from build123d import *

# Parameters (mm, degrees)
SKETCH1_W             = 110
SKETCH1_H             = 46
BOSS_EXTRUDE1_DEPTH   = 6.35
F_8_CLEARANCE_HOLE2_D = 4.3053
FILLET1_R             = 5
M5_CLEARANCE_HOLE1_D  = 5.3
F_8_CLEARANCE_HOLE1_D = 4.3053
SKETCH13_R            = 2.15265
CUT_EXTRUDE2_DEPTH    = 10
CUT_EXTRUDE3_DEPTH    = 7.35


with BuildPart() as part:
    # Sketch1 → Boss-Extrude1 (new body)
    with BuildSketch(Plane.XY):
        Rectangle(SKETCH1_W, SKETCH1_H)
    extrude(amount=BOSS_EXTRUDE1_DEPTH)

    # #8 Clearance Hole2 (through all)
    with Locations(Plane(origin=(0, 0, 0), x_dir=(-1, 0, 0), z_dir=(0, 0, -1))):
        with Locations((-47, 9), (-23, 9), (-23, -9), (-47, -9), (23, -9), (23, 9), (47, 9), (47, -9)):
            Hole(F_8_CLEARANCE_HOLE2_D / 2)

    # Fillet1
    fillet1_edges = [part.edges().sort_by_distance(p)[0] for p in [
        (-55, -23, 3.175),
        (-55, 23, 3.175),
        (55, 23, 3.175),
        (55, -23, 3.175),
    ]]
    fillet(fillet1_edges, radius=FILLET1_R)

    # M5 Clearance Hole1 (through all)
    with Locations(Plane.XY.offset(6.35)):
        with Locations((-10, -5), (10, -5)):
            Hole(M5_CLEARANCE_HOLE1_D / 2)

    # #8 Clearance Hole1 (through all)
    with Locations(Plane.XY.offset(6.35)):
        with Locations((-23, 19), (-23, -19), (23, -19), (23, 19), (-50, 19), (-50, -19), (50, -19), (50, 19)):
            Hole(F_8_CLEARANCE_HOLE1_D / 2)

    # Sketch13 → Cut-Extrude2 (cut)
    with BuildSketch(Plane.XY.offset(6.35)):
        with Locations((47, 9)):
            Circle(SKETCH13_R)
        with Locations((23, -9)):
            Circle(SKETCH13_R)
        with Locations((23, 9)):
            Circle(SKETCH13_R)
        with Locations((47, -9)):
            Circle(SKETCH13_R)
        with BuildLine():
            Line((42, 10), (42, -10))
            ThreePointArc((42, -10), (35, -17), (28, -10))
            Line((28, -10), (28, 10))
            ThreePointArc((28, 10), (35, 17), (42, 10))
        make_face()
        with BuildLine():
            Line((-42, 10), (-42, -10))
            ThreePointArc((-42, -10), (-35, -17), (-28, -10))
            Line((-28, -10), (-28, 10))
            ThreePointArc((-28, 10), (-35, 17), (-42, 10))
        make_face()
    extrude(amount=-CUT_EXTRUDE2_DEPTH, mode=Mode.SUBTRACT)

    # Sketch14 → Cut-Extrude3 (cut, through all)
    with BuildSketch(Plane.XY.offset(6.35)):
        with BuildLine():
            Line((-12.5, -11), (12.5, -11))
            ThreePointArc((12.5, -11), (16.5, -15), (12.5, -19))
            Line((12.5, -19), (-12.5, -19))
            ThreePointArc((-12.5, -19), (-16.5, -15), (-12.5, -11))
        make_face()
        with BuildLine():
            Line((-12.5, 19), (12.5, 19))
            ThreePointArc((12.5, 19), (16.5, 15), (12.5, 11))
            Line((12.5, 11), (-12.5, 11))
            ThreePointArc((-12.5, 11), (-16.5, 15), (-12.5, 19))
        make_face()
    extrude(amount=-CUT_EXTRUDE3_DEPTH, mode=Mode.SUBTRACT)


solid = part.part
The listing builds one solid part. Answer for the finished solid, in the listing's coordinates (mm). A direction names the side the tool comes from. Coordinates: 2 decimals unless noted, no trailing zeros. Loops run counter-clockwise (first coordinate to the right, second up) from the corner with the lowest first, then second, coordinate; pieces in that order, holes last. Notation, with made-up numbers: M -22,-20.75 L -10,-20.75 A23 cw -10,2.25 Z; hole C 0.5,-17 d10. An arc over 180 degrees is marked long. Answer in a Markdown table with one row per item.
1) Determine the mould class of faces 1 (the flat face through (-1, 0, 6.35)), 2 (the cylindrical face through (-54, -21, 3)), 3 (the flat face through (0, -11, 3)), 4 (the cylindrical face through (-16.5, -15.1, 3.2)) for opening direction X: released by +X, released by -X, zero draft, split by the parting line, or undercut.
Answers below:
| item | result |
|---|---|
| face 1 | zero draft |
| face 2 | released by -X |
| face 3 | undercut |
| face 4 | undercut |
2) Find section A-A (x = 35). Determine the outline of the cut face in (y, z).
Answers below:
| item | result |
|---|---|
| outline | M -23,0 L -17,0 L -17,6.35 L -23,6.35 Z; M 17,0 L 23,0 L 23,6.35 L 17,6.35 Z |
3) Find section D-D (y = -14). Determine the outline of the cut face in (x, z).
Answers below:
| item | result |
|---|---|
| outline | M -55,0 L -40.74,0 L -40.74,6.35 L -55,6.35 Z; M -29.26,0 L -16.37,0 L -16.37,6.35 L -29.26,6.35 Z; M 16.37,0 L 29.26,0 L 29.26,6.35 L 16.37,6.35 Z; M 40.74,0 L 55,0 L 55,6.35 L 40.74,6.35 Z |
4) Find section C-C (y = -5). Determine the outline of the cut face in (x, z).
Answers below:
| item | result |
|---|---|
| outline | M -55,0 L -42,0 L -42,6.35 L -55,6.35 Z; M -28,0 L -12.65,0 L -12.65,6.35 L -28,6.35 Z; M -7.35,0 L 7.35,0 L 7.35,6.35 L -7.35,6.35 Z; M 12.65,0 L 28,0 L 28,6.35 L 12.65,6.35 Z; M 42,0 L 55,0 L 55,6.35 L 42,6.35 Z |
5) Find section B-B (x = -23). Determine the outline of the cut face in (y, z).
Answers below:
| item | result |
|---|---|
| outline | M -23,0 L -21.15,0 L -21.15,6.35 L -23,6.35 Z; M -16.85,0 L -11.15,0 L -11.15,6.35 L -16.85,6.35 Z; M -6.85,0 L 6.85,0 L 6.85,6.35 L -6.85,6.35 Z; M 11.15,0 L 16.85,0 L 16.85,6.35 L 11.15,6.35 Z; M 21.15,0 L 23,0 L 23,6.35 L 21.15,6.35 Z |
6) Find the intervals of material crossed by probe 1 along Y at (x, z) = (-23, 3.5); probe 2 along Y at (x, z) = (47, 3.25); probe 3 along Y at (x, z) = (-50, 5.25), in increasing order.
Answers below:
| item | result |
|---|---|
| probe 1 | -23 to -21.15, -16.85 to -11.15, -6.85 to 6.85, 11.15 to 16.85, 21.15 to 23 |
| probe 2 | -23 to -11.15, -6.85 to 6.85, 11.15 to 23 |
| probe 3 | -23 to -21.15, -16.85 to 16.85, 21.15 to 23 |
7) Given pin 1 (4 mm diameter, centred on x = -10, y = -5, fed in from -Z), flat-ended and moving along its own axis, determine where the tip first touches the part or whether it passes through.
Answers below:
| item | result |
|---|---|
| pin 1 | through |
8) Which of the six approach directions +Z, -Z, +X, -X, +Y, -Y give full straight-line access (tool end or side, diameter ignored) to faces 5 (the flat face through (-42, 0, 3)), 6 (the cylindrical face through (53, 22, 3))?
Answers below:
| item | result |
|---|---|
| face 5 | +Z, -Z |
| face 6 | +Z, -Z, +X, +Y |
